Work out the finished part from the listing and answer in its coordinate system (mm). A direction names the side the tool comes from. Give positions to 0.01 mm unless a question says otherwise; leave off trailing zeros. Order: outer loops, then holes, each group sorted by start corner. A loop starts at its lowest first (then second) coordinate and runs counter-clockwise, first axis right, second up. Notation, with made-up numbers: (48, 1) -> (89, 1) arc R20 cw to (89, 6) -> close; hole circle Ø2 at (50.5, 79.5). An arc over 180 degrees is marked (long way). Answer as CSV lines item,"result". Start each with the question number.
1. For faces 1 (the cylindrical face through (-12.91, 1.67, 3.91)), 2 (the flat face through (-10.442, 0, 2)), 3 (the cylindrical face through (-35.3, -0.9, 2.8)), determine the directions among +Z, -Z, +X, -X, +Y, -Y from which every point of the face is accessible in a straight line to the end or side of a thin tool.
2. Flat-ended cylindrical pins translate along their axes: pin 1 (2 mm diameter, centred on x = -19, y = -2.5, fed in from -Z); pin 2 (4 mm diameter, centred on x = -33, z = 0, fed in from -Y). Find the tip coordinate at first contact, or state that the pin passes through.
3. A cutting plane is placed at C-C (x = -29.75). Give the vertices of the cut face in (y, z) (3 decimals).
4. Find the intervals of material crossed by L1, parallel to Y at x = -21.25, z = 0.5; L2, parallel to Y at x = -19.5, z = -1.25; L3, parallel to X at y = -2.75, z = 3.25, in increasing order.
5. A cutting plane is placed at B-B (x = -15.75). Give the vertices of the cut face in (y, z) (3 decimals), then the cut area to 3 significant figures.
6. A cutting plane is placed at A-A (y = 0). Give the vertices of the cut face in (x, z) (3 decimals), then the cut area to 3 significant figures.
from build123d import *

# Parameters (mm, degrees)
SKETCH_1_W   = 5
SKETCH_1_H   = 2.75
SKETCH_1_3_W = 10
SKETCH_1_3_H = 1.401405784
FILLET_1_R   = 10


with BuildPart() as part:
    # 草图1 → 旋转1 (revolve)
    with BuildSketch(Plane(origin=(0, 0, 0), x_dir=(1, 0, 0), z_dir=(0, 1, 0))):
        Polygon((-26.94244556, -1.725), (-15.44244556, -1.725), (-15.44244556, 1.025), (-15.44244556, 2.325), (-26.94244556, 2.325), (-26.94244556, -0.323594216), align=None)
        with Locations((-12.94244556, -0.35)):
            Rectangle(SKETCH_1_W, SKETCH_1_H)
    revolve(axis=Axis((-10.44244556, 0, 1.725), (-1, 0, 0)))

    # 草图1<3> → 旋转2 (revolve)
    with BuildSketch(Plane(origin=(0, 0, 0), x_dir=(1, 0, 0), z_dir=(0, 1, 0))):
        with Locations((-31.94244556, -1.024297108)):
            Rectangle(SKETCH_1_3_W, SKETCH_1_3_H)
    revolve(axis=Axis((-10.44244556, 0, 1.725), (-1, 0, 0)))

    # 圆角1
    # the kernel refuses this fillet: 10 mm, written as the material it adds along each edge
    with BuildSketch(Plane(origin=(-26.94244556, 0, 1.725), x_dir=(0, 0, -1), z_dir=(0, 1, 0))) as fillet_1_piece_1:
        with BuildLine():
            CenterArc((11.401405784, 6.779146923), FILLET_1_R, 180, 42.680903871)
            Line((1.401405784, 6.779146923), (1.201405784, 6.779146923))
            Line((1.201405784, 6.779146923), (1.201405784, 0))
            Line((1.201405784, 0), (1.401405784, -0.2))
            ThreePointArc((1.401405784, -0.2), (2.725702892, -0.2), (3.902971884, -0.135582938))
            Line((3.902971884, -0.135582938), (4.05, 0))
        make_face()
    revolve(axis=Axis((-26.94244556, 0, 1.725), (-1, 0, 0)))


solid = part.part
Answer sheet:
1,face 1,"+X"
1,face 2,"+Z, -Z, +X, +Y, -Y"
1,face 3,"-X"
2,pin 1,"stops at z = -2.04"
2,pin 2,"stops at y = -1.6"
3,outline,"circle Ø4.448 at (0, 1.725)"
4,L1,"y = -3.86 to 3.86"
4,L2,"y = -2.75 to 2.75"
4,L3,"x = -28.08 to -15.44"
5,outline,"circle Ø8.1 at (0, 1.725)"
5,area,"51.5 mm^2"
6,outline,"(-36.942, 0.324) -> (-33.722, 0.324) arc R10 cw to (-26.942, -2.325) -> (-15.442, -2.325) -> (-15.442, -1.025) -> (-10.442, -1.025) -> (-10.442, 4.475) -> (-15.442, 4.475) -> (-15.442, 5.775) -> (-26.942, 5.775) arc R10 cw to (-33.722, 3.126) -> (-36.942, 3.126) -> close"
6,area,"160 mm^2"
